Check sheet for the modelled part. Datum: model origin and axes. Units: mm. A direction names the side the tool comes from. Give positions to 0.01 mm unless a question says otherwise; leave off trailing zeros. Order: outer loops, then holes, each group sorted by start corner. A loop starts at its lowest first (then second) coordinate and runs counter-clockwise, first axis right, second up.
```python
from build123d import *

# Parameters (mm, degrees)
SKETCH1_R                  = 67.5
BOSS_EXTRUDE1_DEPTH        = 10
CUT_EXTRUDE1_DEPTH         = 96.981769102
CUT_EXTRUDE1_DEPTH_BACK    = 96.981769102
SKETCH4_R                  = 4
CUT_EXTRUDE_THIN1_DEPTH    = 96.981769102
F_3_0MM_DOWEL_HOLE1_REACH  = 162.34
F_3_0MM_DOWEL_HOLE1_BORE_R = 1.5
CIRPATTERN1_COUNT          = 4
CUT_EXTRUDE2_DEPTH         = 96.981769113
CUT_EXTRUDE2_DEPTH_BACK    = 3
SKETCH8_R                  = 5


with BuildPart() as part:
    # Sketch1 → Boss-Extrude1 (new body)
    with BuildSketch(Plane(origin=(0, 0, 0), x_dir=(1, 0, 0), z_dir=(0, 1, 0))):
        with Locations(Location((0, 0, 0), (0, 0, 270))):
            Circle(SKETCH1_R)
    extrude(amount=BOSS_EXTRUDE1_DEPTH)

    # Sketch4 → Cut-Extrude1 (cut, two sides: drawn at the far end of the back side and taken through both)
    with BuildSketch(Plane(origin=(0, 10, 0), x_dir=(1, 0, 0), z_dir=(0, 1, 0)).offset(-CUT_EXTRUDE1_DEPTH_BACK)):
        with Locations(Location((-40, 40, 0), (0, 0, 270))):
            Circle(SKETCH4_R)
        with Locations(Location((40, 40, 0), (0, 0, 270))):
            Circle(SKETCH4_R)
        with Locations(Location((40, -40, 0), (0, 0, 270))):
            Circle(SKETCH4_R)
        with Locations(Location((-40, -40, 0), (0, 0, 270))):
            Circle(SKETCH4_R)
    extrude(amount=CUT_EXTRUDE1_DEPTH + CUT_EXTRUDE1_DEPTH_BACK, mode=Mode.SUBTRACT)

    # Sketch5 → Cut-Extrude-Thin1 (cut, through all)
    with BuildSketch(Plane(origin=(0, 10, 0), x_dir=(1, 0, 0), z_dir=(0, 1, 0))):
        Polygon((-31.743671291, 59.570037208), (-59.570037208, 31.743671291), (-66.64110502, 38.814739103), (-38.814739103, 66.64110502), align=None)
        Polygon((59.570037208, 31.743671291), (31.743671291, 59.570037208), (38.814739103, 66.64110502), (66.64110502, 38.814739103), align=None)
        Polygon((31.743671291, -59.570037208), (59.570037208, -31.743671291), (66.64110502, -38.814739103), (38.814739103, -66.64110502), align=None)
        Polygon((-59.570037208, -31.743671291), (-31.743671291, -59.570037208), (-38.814739103, -66.64110502), (-66.64110502, -38.814739103), align=None)
    extrude(amount=-CUT_EXTRUDE_THIN1_DEPTH, mode=Mode.SUBTRACT)

    # Ø3.0mm Dowel Hole1 bore → Ø3.0mm Dowel Hole1 (cut, up to next)
    with BuildSketch(Plane(origin=(45.656854249, 0, 45.656854249), x_dir=(0.7071067811865479, 0, -0.7071067811865471), z_dir=(0.7071067811865471, 0, 0.7071067811865479)), mode=Mode.PRIVATE) as f_3_0mm_dowel_hole1_sk1:
        with Locations((0, 5)):
            Circle(F_3_0MM_DOWEL_HOLE1_BORE_R)
    f_3_0mm_dowel_hole1_tool1 = extrude(f_3_0mm_dowel_hole1_sk1.sketch, amount=-F_3_0MM_DOWEL_HOLE1_REACH, mode=Mode.PRIVATE) & part.part
    f_3_0mm_dowel_hole1 = f_3_0mm_dowel_hole1_tool1.solids().sort_by_distance((45.656854, 5, 45.656854))[0]
    add(f_3_0mm_dowel_hole1, mode=Mode.SUBTRACT)

    # CirPattern1: Ø3.0mm Dowel Hole1 ×4 about axis
    cirpattern1_axis = Axis((0, 10, 0), (0, -1, 0))
    for i in range(1, CIRPATTERN1_COUNT):
        add(f_3_0mm_dowel_hole1.rotate(cirpattern1_axis, i * 360 / CIRPATTERN1_COUNT), mode=Mode.SUBTRACT)

    # Sketch8 → Cut-Extrude2 (cut, two sides: drawn at the far end of the back side and taken through both)
    with BuildSketch(Plane(origin=(0, 10, 0), x_dir=(1, 0, 0), z_dir=(0, 1, 0)).offset(-CUT_EXTRUDE2_DEPTH_BACK)):
        with Locations(Location((0, 0, 0), (0, 0, 90))):
            Circle(SKETCH8_R)
    extrude(amount=CUT_EXTRUDE2_DEPTH + CUT_EXTRUDE2_DEPTH_BACK, mode=Mode.SUBTRACT)


solid = part.part
```
(1) Tool access check on faces 1 (the face through (0, 7, 0)), 2 (the face through (-36.034, 4.93, 39.479)). Record the directions out of +Z, -Z, +X, -X, +Y, -Y that give a thin tool (end or side, any length) a straight path to the whole face; none if there is none.
(2) Sectioned sample at C-C (z = 40). Enter the section's corners in (x, y).
(3) Sectioned sample at A-A (x = 40). Enter the section's corners in (y, z).
(4) Sectioned sample at D-D (x = -2). Enter the section's corners in (y, z).
(5) Release check for a two-part mould opening along X. For faces 3 (the face through (-14, 10, -1)), 4 (the face through (-36.627, 4.93, -37.85)), 5 (the face through (45.462, 7.292, 45.852)) record: released by +X, released by -X, zero draft, split by the parting line, or undercut.
(6) Thickness scan on L1, parallel to X at y = 6.5, z = 40; L2, parallel to Z at x = 39, y = 5. Record the ranges inside material, lowest first.
(7) Go/stop test with flat-tipped pins: P1, Ø1.5, axis at y = 6, z = -47.5, coming from the +X side; P2, Ø5, axis at y = 1.5, z = -30.5, coming from the -X side; P3, Ø5, axis at x = -20, y = 5.5, coming from the +Z side; P4, Ø6.5, axis at x = 40, z = -40, coming from the +Y side. Record where each tip stops, or that it passes through.
(8) Sectioned sample at B-B (z = 0). Enter the section's corners in (x, y), plus the area to 3 significant figures.
Values follow:
1. face 1: +Y
1. face 2: +Y, -Y
2. outline: (-51.31, 0) - (-44, 0) - (-44, 10) - (-51.31, 10) - close; (-36, 0) - (36, 0) - (36, 10) - (-36, 10) - close; (44, 0) - (51.31, 0) - (51.31, 10) - (44, 10) - close
3. outline: (0, -51.31) - (10, -51.31) - (10, -44) - (0, -44) - close; (0, -36) - (10, -36) - (10, 36) - (0, 36) - close; (0, 44) - (10, 44) - (10, 51.31) - (0, 51.31) - close
4. outline: (0, -67.47) - (10, -67.47) - (10, -4.58) - (7, -4.58) - (7, 4.58) - (10, 4.58) - (10, 67.47) - (0, 67.47) - close
5. face 3: zero draft
5. face 4: undercut
5. face 5: released by +X
6. L1: x = -51.31 to -44, -36 to 36, 44 to 51.31
6. L2: z = -52.31 to -43.87, -36.13 to 36.13, 43.87 to 52.31
7. P1: stops at x = 44.56
7. P2: stops at x = -61.42
7. P3: stops at z = 65.19
7. P4: passes through
8. outline: (-67.5, 0) - (67.5, 0) - (67.5, 10) - (5, 10) - (5, 7) - (-5, 7) - (-5, 10) - (-67.5, 10) - close
8. area: 1,320 mm2
